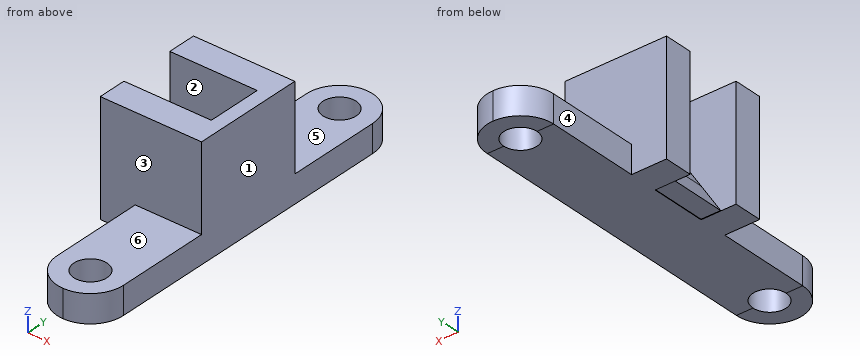
from build123d import *

# Parameters (mm, degrees)
F0_W      = 51
F0_H      = 15
F1_DEPTH  = 36
F3_R      = 9
F4_DEPTH  = 103.1
F6_DEPTH  = 15
F7_DEPTH  = 15
F2_W      = 19
F2_H      = 15.5
F8_DEPTH  = 61
F9_DEPTH  = 100
F10_DEPTH = 100
F11_DEPTH = 25
F12_DEPTH = 25


with BuildPart() as f1:
    # F0 (on Right) → F1 (new body)
    with BuildSketch(Plane.YZ):
        Polygon((30.5, 30.5), (-30.5, 30.5), (-30.5, -15.5), (-30.5, -30.5), (30.5, -30.5), (30.5, -15.5), align=None)
        with Locations((-56, -23)):
            Rectangle(F0_W, F0_H)
        with Locations((56, -23)):
            Rectangle(F0_W, F0_H)
        Polygon((-81.5, -30.5), (-81.5, -15.5), (-99.5, -15.5), (-99.5, -30.6042674929), align=None)
        Polygon((99.5, -15.5), (81.5, -15.5), (81.5, -30.5), (99.5, -30.6042674929), align=None)
    extrude(amount=F1_DEPTH)

    # F3 (on Top) → F4 (cut)
    with BuildSketch(Plane.XY):
        with Locations((18, 81.5)):
            Circle(F3_R)
        with Locations((18, -81.5)):
            Circle(F3_R)
    extrude(amount=-F4_DEPTH, mode=Mode.SUBTRACT)

    # F5 (on Front) → F6 (cut)
    with BuildSketch(Plane.XZ):
        Polygon((0, -13.7268389231), (28.6131525338, 30.7420096008), (-18.6368474662, 30.7420096008), (-18.6368474662, -30.2579903992), (-10.6368474662, -30.2579903992), align=None)
    extrude(amount=F6_DEPTH, mode=Mode.SUBTRACT)

    # F5 (on Front) → F7 (cut)
    with BuildSketch(Plane.XZ):
        Polygon((0, -13.7268389231), (28.6131525338, 30.7420096008), (-18.6368474662, 30.7420096008), (-18.6368474662, -30.2579903992), (-10.6368474662, -30.2579903992), align=None)
    extrude(amount=-F7_DEPTH, mode=Mode.SUBTRACT)

    # F2 (on face) → F8 (join)
    with BuildSketch(Plane.XY.offset(30.5)):
        with Locations((-9.5, 22.75)):
            Rectangle(F2_W, F2_H)
        with Locations((-9.5, -22.75)):
            Rectangle(F2_W, F2_H)
    extrude(amount=-F8_DEPTH)

    # F2 (on face) → F9 (cut)
    with BuildSketch(Plane.XY.offset(30.5)):
        with BuildLine():
            Line((36, -99.5), (36, -81.5))
            ThreePointArc((36, -81.5), (30.7279220614, -94.2279220614), (18, -99.5))
            Line((18, -99.5), (36, -99.5))
        make_face()
        with BuildLine():
            ThreePointArc((18, 99.5), (30.7279220614, 94.2279220614), (36, 81.5))
            Line((36, 81.5), (36, 99.5))
            Line((36, 99.5), (18, 99.5))
        make_face()
        with BuildLine():
            Line((0, 99.5), (0, 81.4999998705))
            ThreePointArc((0, 81.4999998705), (5.2720778928, 94.2279220156), (18, 99.5))
            Line((18, 99.5), (0, 99.5))
        make_face()
    extrude(amount=-F9_DEPTH, mode=Mode.SUBTRACT)

    # F2 (on face) → F10 (cut)
    with BuildSketch(Plane.XY.offset(30.5)):
        with BuildLine():
            ThreePointArc((18, -99.5), (5.2720779386, -94.2279220614), (0, -81.5))
            Line((0, -81.5), (0, -99.5))
            Line((0, -99.5), (18, -99.5))
        make_face()
        with BuildLine():
            Line((36, -99.5), (36, -81.5))
            ThreePointArc((36, -81.5), (30.7279220614, -94.2279220614), (18, -99.5))
            Line((18, -99.5), (36, -99.5))
        make_face()
    extrude(amount=-F10_DEPTH, mode=Mode.SUBTRACT)

    # F5 (on Front) → F11 (join)
    with BuildSketch(Plane.XZ):
        Polygon((0, -30.2579903992), (0, -13.7268389231), (-10.6368474662, -30.2579903992), align=None)
    extrude(amount=F11_DEPTH)

    # F5 (on Front) → F12 (join)
    with BuildSketch(Plane.XZ):
        Polygon((0, -30.2579903992), (0, -13.7268389231), (-10.6368474662, -30.2579903992), align=None)
    extrude(amount=-F12_DEPTH)


solid = f1.part
Input: part model. Units: mm. Frame: model coordinates. Face numbers are marked on the shaded views. A direction names the side the tool comes from. Round coordinates to 2 decimals unless told otherwise and drop trailing zeros. Order: outer loops, then holes, each group sorted by start corner. A loop starts at its lowest first (then second) coordinate and runs counter-clockwise, first axis right, second up. Notation, with made-up numbers: (-20.5, 35.25) - (-10.5, 35.25) arc R7 cw to (-10.5, 40.25) - close; hole circle Ø6 at (31, 20.25). An arc over 180 degrees is marked (long way). Answer as a JSON object with one key per item and string values. Group by question number.
(1) Cut plane A-A (x = 23). Return loops of the section in (y, z).
(2) Cut plane C-C (x = 4.5). Return loops of the section in (y, z).
(3) Cut plane D-D (x = 12.5). Return loops of the section in (y, z).
(4) Draft query along Y for the marked faces 1, 2 and 3. Return one class per face: released by +Y, released by -Y, zero draft, split by the parting line, or undercut.
(5) Cut plane B-B (z = -3). Return loops of the section in (x, y).
(6) Reachability of the marked faces 4, 5 and 6 from +Z, -Z, +X, -X, +Y, -Y: full face, straight path, thin tool, end or side. Return the list, or none.
(7) Material intervals for probe 1 along Y at (x, z) = (18, -23.75); probe 2 along Y at (x, z) = (3.5, -5.5); probe 3 along X at (y, z) = (-81.5, -23.75), sorted ascending. Write a range as from..to.
(8) Pin query (flat end, axial travel): P1, Ø12, axis at y = 70.5, z = -17.5, coming from the -X side; P2, Ø4, axis at x = 4.5, z = 0.5, coming from the +Y side; P3, Ø11.5, axis at x = -6, y = -7, coming from the -Z side. Return the tip coordinate at first contact, or that it passes through.
Here are the results:
{
 "1": {"outline": "(-98.79, -30.6) - (-88.98, -30.54) - (-88.98, -15.5) - (-98.79, -15.5) - close; (-74.02, -30.5) - (74.02, -30.5) - (74.02, -15.5) - (30.5, -15.5) - (30.5, 30.5) - (15, 30.5) - (15, 22.02) - (-15, 22.02) - (-15, 30.5) - (-30.5, 30.5) - (-30.5, -15.5) - (-74.02, -15.5) - close; (88.98, -30.54) - (98.79, -30.6) - (98.79, -15.5) - (88.98, -15.5) - close"},
 "2": {"outline": "(-93.41, -30.57) - (-81.5, -30.5) - (81.5, -30.5) - (93.41, -30.57) - (93.41, -15.5) - (30.5, -15.5) - (30.5, 30.5) - (15, 30.5) - (15, -6.73) - (-15, -6.73) - (-15, 30.5) - (-30.5, 30.5) - (-30.5, -15.5) - (-93.41, -15.5) - close"},
 "3": {"outline": "(-98.64, -30.6) - (-88.62, -30.54) - (-88.62, -15.5) - (-98.64, -15.5) - close; (-74.38, -30.5) - (74.38, -30.5) - (74.38, -15.5) - (30.5, -15.5) - (30.5, 30.5) - (15, 30.5) - (15, 5.7) - (-15, 5.7) - (-15, 30.5) - (-30.5, 30.5) - (-30.5, -15.5) - (-74.38, -15.5) - close; (88.62, -30.54) - (98.64, -30.6) - (98.64, -15.5) - (88.62, -15.5) - close"},
 "4": {"face 1": "zero draft", "face 2": "undercut", "face 3": "released by -Y"},
 "5": {"outline": "(-19, -30.5) - (36, -30.5) - (36, 30.5) - (-19, 30.5) - (-19, 15) - (6.9, 15) - (6.9, -15) - (-19, -15) - close"},
 "6": {"face 4": "+Z, -Z, -X, +Y", "face 5": "+Z, +X, -X, +Y", "face 6": "+Z, +X, -X, -Y"},
 "7": {"probe 1": "y = -99.5..-90.5, -72.5..72.5, 90.5..99.5", "probe 2": "y = -30.5..-15, 15..30.5", "probe 3": "x = 0..9, 27..36"},
 "8": {"P1": "stops at x = 0", "P2": "stops at y = 30.5", "P3": "stops at z = -30.26"}
}
